Here's the drawing with two shaded views (mm, measured from the low corner). I have some questions. Give positions to 0.01 mm unless a question says otherwise; leave off trailing zeros. Write each loop counter-clockwise with the first axis right and the second up, starting at its lowest first coordinate (ties: lowest second). Pieces come first, ordered by that corner, then holes. Notation, with made-up numbers: (-13, 74.5) -> (19, 74.5) arc R25 cw to (19, 96.5) -> close; hole circle Ø10 at (13, 89). An arc over 180 degrees is marked (long way). One line per item, written item: value.
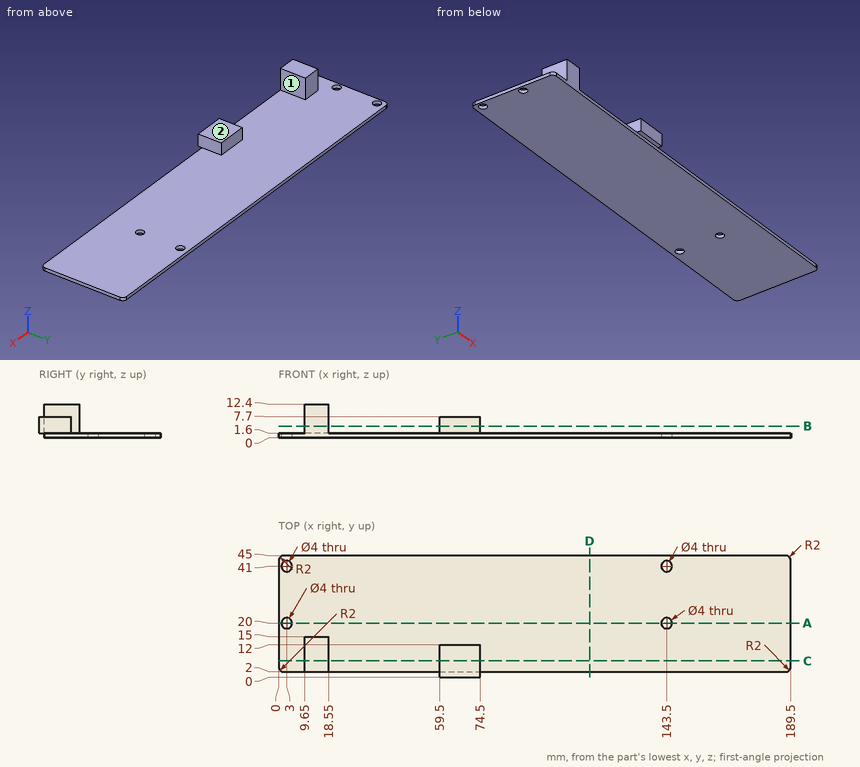
1) If we section it at B-B (z = 4.25): Write out the boundary of the cut face in (x, y), and give its area (3 significant figures).
Answer list:
outline: (9.65, 2) -> (18.55, 2) -> (18.55, 15) -> (9.65, 15) -> close; (59.5, 0) -> (74.5, 0) -> (74.5, 12) -> (59.5, 12) -> close
area: 296 mm^2
2) If we section it at C-C (y = 6): Write out the boundary of the cut face in (x, z), and give its area (3 significant figures).
Answer list:
outline: (0, 0) -> (189.5, 0) -> (189.5, 1.6) -> (74.5, 1.6) -> (74.5, 7.7) -> (59.5, 7.7) -> (59.5, 1.6) -> (18.55, 1.6) -> (18.55, 12.4) -> (9.65, 12.4) -> (9.65, 1.6) -> (0, 1.6) -> close
area: 491 mm^2
3) I need wall thicknesses on L1, parallel to Y at x = 3, z = 0.65; L2, parallel to Z at x = 76, y = 22; L3, parallel to X at y = 13, z = 3.5. Which ranges of each line are inside material? Lowest first, please.
Answer list:
L1: y = 2 to 18, 22 to 39, 43 to 45
L2: z = 0 to 1.6
L3: x = 9.65 to 18.55
4) If we section it at D-D (x = 115): Write out the boundary of the cut face in (y, z), and give its area (3 significant figures).
Answer list:
outline: (2, 0) -> (45, 0) -> (45, 1.6) -> (2, 1.6) -> close
area: 68.8 mm^2
5) If we section it at A-A (y = 20): Write out the boundary of the cut face in (x, z), and give its area (3 significant figures).
Answer list:
outline: (0, 0) -> (1, 0) -> (1, 1.6) -> (0, 1.6) -> close; (5, 0) -> (141.5, 0) -> (141.5, 1.6) -> (5, 1.6) -> close; (145.5, 0) -> (189.5, 0) -> (189.5, 1.6) -> (145.5, 1.6) -> close
area: 290 mm^2
6) Will these pins go through, and if not, where does the flat tip stop? pin 1 (3 mm diameter, centred on x = 64.5, z = 4.5, fed in from +Y); pin 2 (5 mm diameter, centred on x = 3, y = 20, fed in from +Z); pin 3 (1.8 mm diameter, centred on y = 7, z = 5, fed in from +X); pin 4 (2.5 mm diameter, centred on x = 143.5, y = 20, fed in from +Z).
Answer list:
pin 1: stops at y = 12
pin 2: stops at z = 1.6
pin 3: stops at x = 74.5
pin 4: passes through
7) We'd pull the mould along X, two halves only. Please class the marked faces 1 and 2: released by +X, released by -X, zero draft, split by the parting line, or undercut.
Answer list:
face 1: undercut
face 2: zero draft
